from build123d import *

# Parameters (mm, degrees)
BOSS_EXTRU_1_DEPTH = 7


with BuildPart() as part:
    # Esquisse1 → Révolution1 (revolve)
    with BuildSketch(Plane.XY):
        Polygon((-4, 0), (-4, 18), (-2, 18), (-2, 25), (-9.5, 25), (-9.5, 0), align=None)
    revolve(axis=Axis((0, 0, 0), (0, -1, 0)))

    # Esquisse2 → Boss.-Extru.1 (add)
    with BuildSketch(Plane(origin=(0, 25, 0), x_dir=(1, 0, 0), z_dir=(0, 1, 0))):
        with BuildLine():
            Line((-1.322875656, 1.5), (1.322875656, 1.5))
            ThreePointArc((1.322875656, 1.5), (0, 2), (-1.322875656, 1.5))
        make_face()
    extrude(amount=-BOSS_EXTRU_1_DEPTH)


solid = part.part
Work out the finished part from the listing and answer in its coordinate system (mm). A direction names the side the tool comes from. Give positions to 0.01 mm unless a question says otherwise; leave off trailing zeros. Write each loop counter-clockwise with the first axis right and the second up, starting at its lowest first coordinate (ties: lowest second). Pieces come first, ordered by that corner, then holes. Notation, with made-up numbers: (28, 71.25) - (32, 71.25) arc R10 cw to (32, 83.25) - close; hole circle Ø5 at (-34.75, 77.25). An arc over 180 degrees is marked (long way). One line per item, written item: value. Start each with the question number.
1. For faces 1 (the flat face through (0, 22, -1.5)), 2 (the flat face through (-2, 0, 4)), 3 (the cylindrical face through (0.867, 9.126, 3.905)), determine the directions among +Z, -Z, +X, -X, +Y, -Y from which every point of the face is accessible in a straight line to the end or side of a thin tool.
2. Find section D-D (z = -2.5). Write down the section's boundary in (x, y).
3. For a pull along Z with two mould halves and no side action, classify faces 4 (the cylindrical face through (0, 22, 2)), 5 (the flat face through (0, 18, -2)), 6 (the flat face through (0, 25, -2)), 7 (the cylindrical face through (-4.38, 12.32, 8.43)) as +Z half, -Z half, draft (parallel to the pull), parting line (faces both ways), or undercut.
4. Consider probe 1 along X at (y, z) = (14, 0); probe 2 along X at (y, z) = (22.5, 0). Determine where each line is inside the solid, lowest interval first.
5. Find section A-A (z = 0). Write down the section's boundary in (x, y), then the cut area to 3 significant figures.
6. Find section C-C (y = 20.5). Write down the section's boundary in (x, z).
7. Find section B-B (x = 0). Write down the section's boundary in (y, z).
8. Given pin 1 (4 mm diameter, centred on x = 5.5, y = 17, fed in from +Z); pin 2 (3.5 mm diameter, centred on x = 0, z = 0, fed in from -Y); pin 3 (1.5 mm diameter, centred on x = 3.5, y = 8.5, fed in from -Z), each flat-ended and moving along its own axis, determine where each tip first touches the part or whether it passes through.
Geometry results:
1. face 1: +Y, -Y
1. face 2: +Z, -Z, +X, -X, -Y
1. face 3: -Y
2. outline: (-9.17, 0) - (-3.12, 0) - (-3.12, 18) - (3.12, 18) - (3.12, 0) - (9.17, 0) - (9.17, 25) - (-9.17, 25) - close
3. face 4: undercut
3. face 5: undercut
3. face 6: draft
3. face 7: parting line
4. probe 1: -9.5 to -4, 4 to 9.5
4. probe 2: -9.5 to -2, 2 to 9.5
5. outline: (-9.5, 0) - (-4, 0) - (-4, 18) - (-2, 18) - (-2, 25) - (-9.5, 25) - close; (2, 18) - (4, 18) - (4, 0) - (9.5, 0) - (9.5, 25) - (2, 25) - close
5. area: 303 mm2
6. outline: circle Ø19 at (0, 0); hole (-1.32, -1.5) - (1.32, -1.5) arc R2 ccw (long way) to start
7. outline: (0, -9.5) - (25, -9.5) - (25, -1.5) - (18, -1.5) - (18, -4) - (0, -4) - close; (0, 4) - (18, 4) - (18, 2) - (25, 2) - (25, 9.5) - (0, 9.5) - close
8. pin 1: z = 8.83
8. pin 2: y = 18
8. pin 3: z = -9.09
